Source: CAD feature listing. Evaluate the final solid. Frame: model axes, mm. Face numbers are marked on the shaded views. A direction names the side the tool comes from. Give positions to 0.01 mm unless a question says otherwise; leave off trailing zeros. Loops run counter-clockwise (first coordinate to the right, second up) from the corner with the lowest first, then second, coordinate; pieces in that order, holes last. Notation, with made-up numbers: M 79,41 L 84,41 A26 cw 84,59 Z; hole C 31.25,-6 d8. An arc over 180 degrees is marked long. Answer in a Markdown table with one row per item.
```python
from build123d import *

# Parameters (mm, degrees)
F0_W     = 70
F0_H     = 37
F1_DEPTH = 41.5
F2_DEPTH = 35.5
F3_W     = 80
F3_H     = 26.6440417618
F3_W_2   = 40
F4_DEPTH = 40


with BuildPart() as f1:
    # F0 (on Top) → F1 (new body)
    with BuildSketch(Plane.XY):
        with Locations((-35, 0)):
            Rectangle(F0_W, F0_H)
    extrude(amount=F1_DEPTH)

    # F0 (on Top) → F2 (join)
    with BuildSketch(Plane.XY):
        with Locations((35, 0)):
            Rectangle(F0_W, F0_H)
        with Locations((-35, 0)):
            Rectangle(F0_W, F0_H)
    extrude(amount=F2_DEPTH)

    # F3 (on face) → F4 (cut)
    with BuildSketch(Plane(origin=(0, 18.5, 0), x_dir=(-1, 0, 0), z_dir=(0, 1, 0))):
        with Locations((20, 13.3220208809)):
            Rectangle(F3_W, F3_H)
        with Locations((-50, 13.3220208809)):
            Rectangle(F3_W_2, F3_H)
    extrude(amount=-F4_DEPTH, mode=Mode.SUBTRACT)


solid = f1.part
```
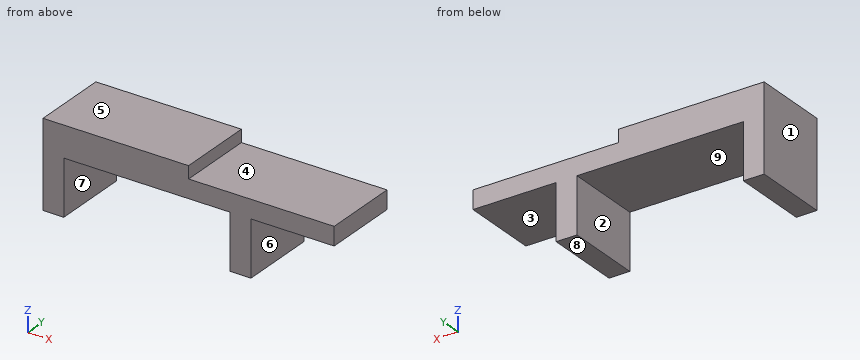
Q1. Section query C-C (x = 54). Output: boundary loops of the cut face in (y, z).
Values follow:
| item | result |
|---|---|
| outline | M -18.5,26.64 L 18.5,26.64 L 18.5,35.5 L -18.5,35.5 Z |
Q2. Reachability of the marked faces 1, 2, 3, 4 and 5 from +Z, -Z, +X, -X, +Y, -Y: full face, straight path, thin tool, end or side. Return the list, or none.
Values follow:
| item | result |
|---|---|
| face 1 | +Z, -Z, -X, +Y, -Y |
| face 2 | -Z, +Y, -Y |
| face 3 | -Z, +X, +Y, -Y |
| face 4 | +Z, +X, +Y, -Y |
| face 5 | +Z, +X, -X, +Y, -Y |
Q3. Section query B-B (y = 6). Output: boundary loops of the cut face in (x, z), plus the area to 3 significant figures.
Values follow:
| item | result |
|---|---|
| outline | M -70,0 L -60,0 L -60,26.64 L 20,26.64 L 20,0 L 30,0 L 30,26.64 L 70,26.64 L 70,35.5 L 0,35.5 L 0,41.5 L -70,41.5 Z |
| area | 2,190 mm^2 |
Q4. Contact query for flat-ended pins moving along their axis: pin 1 Ø1 at (x, y) = (-17, -10) entering from -Z; pin 2 Ø4 at (x, y) = (16.5, 6.5) entering from +Z; pin 3 Ø5 at (y, z) = (-3.5, 8.5) entering from +X. Output: stop coordinate, or through.
Values follow:
| item | result |
|---|---|
| pin 1 | z = 26.64 |
| pin 2 | z = 35.5 |
| pin 3 | x = 30 |
Q5. Ray query, probe 1 along X at (y, z) = (-15, 12.5); probe 2 along Z at (x, y) = (63.5, 6); probe 3 along X at (y, z) = (-3, 38.5). Return the intervals inside material, ascending. Write a range as from..to.
Values follow:
| item | result |
|---|---|
| probe 1 | -70..-60, 20..30 |
| probe 2 | 26.64..35.5 |
| probe 3 | -70..0 |
Q6. Section query D-D (x = 26.5). Output: boundary loops of the cut face in (y, z), plus the area to 3 significant figures.
Values follow:
| item | result |
|---|---|
| outline | M -18.5,0 L 18.5,0 L 18.5,35.5 L -18.5,35.5 Z |
| area | 1,310 mm^2 |
Q7. Mould query, pull axis X, two halves, no side actions, for the marked faces 6, 7, 8 and 9. Classes: +X half, -X half, draft (parallel to the pull), parting line (faces both ways), or undercut.
Values follow:
| item | result |
|---|---|
| face 6 | +X half |
| face 7 | undercut |
| face 8 | draft |
| face 9 | undercut |
Q8. Section query A-A (z = 21). Output: boundary loops of the cut face in (x, y).
Values follow:
| item | result |
|---|---|
| outline | M -70,-18.5 L -60,-18.5 L -60,18.5 L -70,18.5 Z; M 20,-18.5 L 30,-18.5 L 30,18.5 L 20,18.5 Z |
